Here's how the part is built. I have some questions about the finished solid (model axes, mm). Coordinates: 2 decimals unless noted, no trailing zeros. Order: outer loops, then holes, each group sorted by start corner. A loop starts at its lowest first (then second) coordinate and runs counter-clockwise, first axis right, second up. Notation, with made-up numbers: (45, 12.25) - (60, 12.25) arc R12 cw to (60, 23.25) - close; hole circle Ø2 at (-25.75, -30.75). An arc over 180 degrees is marked (long way). Answer as CSV lines item,"result". Start each with the question number.
Item 1: Imagine slicing it at C-C on z = 6.5. List the corners of the cut face in (x, y) for me.
Item 2: Imagine slicing it at A-A on y = 0. List the corners of the cut face in (x, z) for me, and give its area (3 significant figures).
Item 3: I'm going to push a flat-ended pin straight in: pin 1 (3 mm diameter, centred on y = 1, z = -11.5, fed in from +X). Where does the tip first touch, or does it pass through?
Item 4: I need wall thicknesses on line 1 (X direction, y = -1.3, z = 0.5); line 2 (Z direction, x = 117, y = 1.95); line 3 (Z direction, x = 23.5, y = -0.2). Which ranges of each line are inside material? Lowest first, please.
from build123d import *

# Parameters (mm, degrees)
F0_W     = 5
F0_H     = 45
F1_DEPTH = 120
F2_SIZE  = 4.99999
F3_R     = 0.8
F4_DEPTH = 2.5
F5_R     = 0.8
F6_DEPTH = 2.5


# Not quite as in the source:
# - a fillet or chamfer is up to 0.001 mm smaller than in the source, because OpenCascade refuses the exact size


with BuildPart() as f1:
    # F0 (on Right) → F1 (new body)
    with BuildSketch(Plane.YZ):
        Rectangle(F0_W, F0_H)
    extrude(amount=F1_DEPTH)

    # F2 (size 5 in the source; OpenCascade refuses exactly that, so slightly less here)
    f2_edges = [f1.edges().sort_by_distance(p)[0] for p in [
        (60, -2.5, -22.5),
    ]]
    chamfer(f2_edges, length=F2_SIZE)

    # F3 (on face) → F4 (join)
    with BuildSketch(Plane(origin=(0, 0, 0), x_dir=(0, -1, 0), z_dir=(-1, 0, 0))):
        Circle(F3_R)
    extrude(amount=F4_DEPTH)

    # F5 (on face) → F6 (join)
    with BuildSketch(Plane.YZ.offset(120)):
        Circle(F5_R)
    extrude(amount=F6_DEPTH)


solid = f1.part
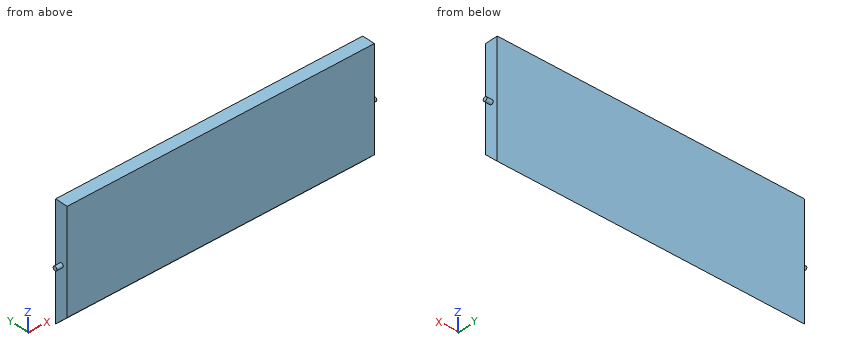
Responses:
1,outline,"(0, -2.5) - (120, -2.5) - (120, 2.5) - (0, 2.5) - close"
2,outline,"(-2.5, -0.8) - (0, -0.8) - (0, -20) - (120, -20) - (120, -0.8) - (122.5, -0.8) - (122.5, 0.8) - (120, 0.8) - (120, 22.5) - (0, 22.5) - (0, 0.8) - (-2.5, 0.8) - close"
2,area,"5,110 mm^2"
3,pin 1,"stops at x = 120"
4,line 1,"x = 0 to 120"
4,line 2,"z = -21.95 to 22.5"
4,line 3,"z = -19.8 to 22.5"
